Source: three-view drawing plus pictorial views. Frame: mm from the lowest corner of the part. A direction names the side the tool comes from. Give positions to 0.01 mm unless a question says otherwise; leave off trailing zeros. Order: outer loops, then holes, each group sorted by start corner. A loop starts at its lowest first (then second) coordinate and runs counter-clockwise, first axis right, second up.
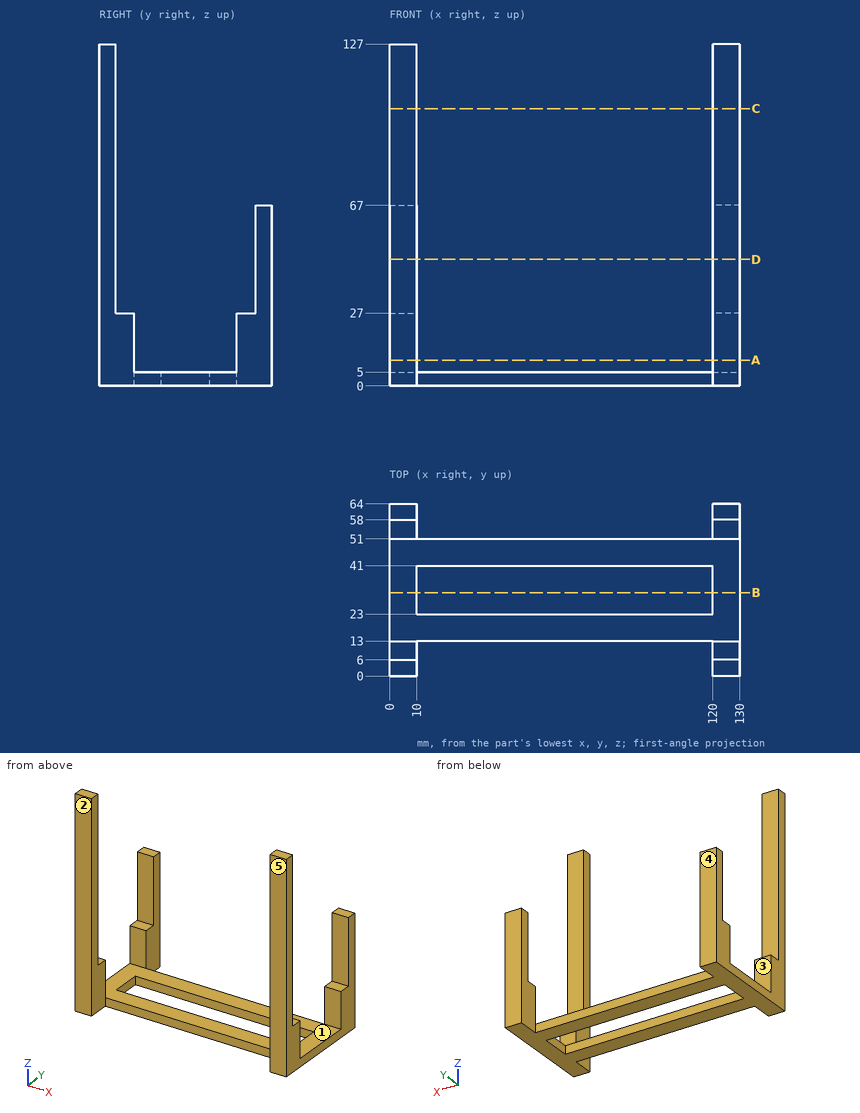
(1) Section A-A, the plane z = 9.5. Return loops of the section in (x, y).
(2) Section B-B, the plane y = 31. Return loops of the section in (x, z).
(3) Line query: line 1 along X through (y, z) = (59, 11); line 2 along Y through (x, z) = (8.5, 19.5); line 3 along Z through (x, y) = (15, 22.5). Output: solid intervals per line, ascending.
(4) Section D-D, the plane z = 47. Return loops of the section in (x, y), plus the area to 3 significant figures.
(5) Section C-C, the plane z = 103. Return loops of the section in (x, y).
(6) Access query for the marked faces 1 and 2. Directions: +Z, -Z, +X, -X, +Y, -Y. A direction counts if a zero-diameter tool reaches every point of the face in a straight line with its end or side. Return the directions, or none.
(7) Draft query along Y for the marked faces 3, 4 and 5. Return one class per face: +Y half, -Y half, draft (parallel to the pull), parting line (faces both ways), or undercut.
(8) Pin query (flat end, axial travel): pin 1 Ø3 at (x, y) = (102.5, 38.5) entering from -Z; pin 2 Ø3 at (x, y) = (3, 61.5) entering from +Z; pin 3 Ø5.5 at (x, z) = (39.5, 1.5) entering from -Y. Return the tip coordinate at first contact, or that it passes through.
Checks:
1. outline: (0, 0) - (10, 0) - (10, 13) - (0, 13) - close; (0, 51) - (10, 51) - (10, 64) - (0, 64) - close; (120, 0) - (130, 0) - (130, 13) - (120, 13) - close; (120, 51) - (130, 51) - (130, 64) - (120, 64) - close
2. outline: (0, 0) - (10, 0) - (10, 5) - (0, 5) - close; (120, 0) - (130, 0) - (130, 5) - (120, 5) - close
3. line 1: x = 0 to 10, 120 to 130
3. line 2: y = 0 to 13, 51 to 64
3. line 3: z = 0 to 5
4. outline: (0, 0) - (10, 0) - (10, 6) - (0, 6) - close; (0, 58) - (10, 58) - (10, 64) - (0, 64) - close; (120, 0) - (130, 0) - (130, 6) - (120, 6) - close; (120, 58) - (130, 58) - (130, 64) - (120, 64) - close
4. area: 240 mm2
5. outline: (0, 0) - (10, 0) - (10, 6) - (0, 6) - close; (120, 0) - (130, 0) - (130, 6) - (120, 6) - close
6. face 1: +Z, +X, -X
6. face 2: +Z, -Z, +X, -X, -Y
7. face 3: undercut
7. face 4: +Y half
7. face 5: -Y half
8. pin 1: passes through
8. pin 2: stops at z = 67
8. pin 3: stops at y = 13
